The listing builds one solid part. Answer for the finished solid, in the listing's coordinates (mm). A direction names the side the tool comes from. Coordinates: 2 decimals unless noted, no trailing zeros. Loops run counter-clockwise (first coordinate to the right, second up) from the corner with the lowest first, then second, coordinate; pieces in that order, holes last. Notation, with made-up numbers: (-13.5, 24) - (42.5, 24) arc R35 cw to (42.5, 62) - close; hole circle Ø5 at (29.25, 21.25). An arc over 180 degrees is marked (long way). Return JSON: item names as keys, results as strings. Group by question number.
1. Each of these flat-tipped pins is pushed along its axis until it touches: P1, Ø4, axis at x = -6.5, y = -1.5, coming from the +Z side; P2, Ø1, axis at x = -4.5, y = -3.5, coming from the +Z side; P3, Ø3, axis at y = -1, z = -6.5, coming from the +X side (3 decimals). Where does it stop, or does it pass through?
2. Section B-B (z = 15.5) is taken. Write down the section's boundary in (x, y), and give its area (3 significant figures).
3. Find the intervals of material crossed by line 1 along Z through (x, y) = (2.5, -4.5); line 2 along Z through (x, y) = (-6.75, -6.5); line 3 along X through (y, z) = (-2.75, -3), in increasing order.
4. Which of the six approach directions +Z, -Z, +X, -X, +Y, -Y give full straight-line access (tool end or side, diameter ignored) to faces 1 (the face through (-1.037, -3.451, 14.204)), 2 (the face through (-8.336, -3.451, 16.078))?
5. Section C-C (x = 11.75) is taken. Write down the section's boundary in (y, z), and give its area (3 significant figures).
6. Section A-A (y = -2.75) is taken. Write down the section's boundary in (x, z) (3 decimals).
7. The mould has two halves that part along Z. Classify faces 3 (the face through (-0.07, 0, 10.03)), 4 (the face through (8.513, -3.451, 16.027)), 5 (the face through (-1.924, -3.465, -8.664)): pulls with the +Z half, pulls with the -Z half, needs draft (parallel to the pull), parting line crosses it, or undercut.
```python
from build123d import *

# Parameters (mm, degrees)
F0_R     = 8.875
F1_DEPTH = 7
F2_SIZE  = 1


with BuildPart() as f1:
    # F0 (on Front) → F1 (new body)
    with BuildSketch(Plane.XZ):
        with BuildLine():
            ThreePointArc((0, 10.625), (7.51301, 7.51301), (10.625, 0))
            Line((10.625, 0), (14.745765, 14.220767))
            Line((14.745765, 14.220767), (2.103486, 17.884132))
            Line((2.103486, 17.884132), (0, 10.625))
        make_face()
        with BuildLine():
            ThreePointArc((-10.625, 0), (-7.51301, 7.51301), (0, 10.625))
            Line((0, 10.625), (-2.103486, 17.884132))
            Line((-2.103486, 17.884132), (-14.745765, 14.220767))
            Line((-14.745765, 14.220767), (-10.625, 0))
        make_face()
        with BuildLine():
            ThreePointArc((-10.625, 0), (0, -10.625), (10.625, 0))
            ThreePointArc((10.625, 0), (7.51301, 7.51301), (0, 10.625))
            ThreePointArc((0, 10.625), (-7.51301, 7.51301), (-10.625, 0))
        make_face()
        Circle(F0_R, mode=Mode.SUBTRACT)
    extrude(amount=F1_DEPTH)

    # F2
    f2_edges = [f1.edges().sort_by_distance(p)[0] for p in [
        (-8.875, 0, 0),
        (-8.875, -7, 0),
    ]]
    chamfer(f2_edges, length=F2_SIZE)


solid = f1.part
```
The answers:
{
 "1": {"P1": "stops at z = 17.19", "P2": "stops at z = 17.33", "P3": "stops at x = 9.375"},
 "2": {"outline": "(-10.33, -7) - (-1.41, -7) - (-1.41, 0) - (-10.33, 0) - close; (1.41, -7) - (10.33, -7) - (10.33, 0) - (1.41, 0) - close", "area": "125 mm2"},
 "3": {"line 1": "z = -10.33 to -8.52, 8.52 to 17.77", "line 2": "z = -8.21 to -6.51, 6.51 to 16.54", "line 3": "x = -10.19 to -8.35, 8.35 to 10.19"},
 "4": {"face 1": "+Z, +Y, -Y", "face 2": "+Z, -X, +Y, -Y"},
 "5": {"outline": "(-7, 3.88) - (0, 3.88) - (0, 15.09) - (-7, 15.09) - close", "area": "78.4 mm2"},
 "6": {"outline": "(-14.746, 14.221) - (-10.625, 0) arc R10.625 ccw to (10.625, 0) - (14.746, 14.221) - (2.103, 17.884) - (0, 10.625) - (-2.103, 17.884) - close; hole circle Ø17.75 at (0, 0)"},
 "7": {"face 3": "needs draft", "face 4": "pulls with the +Z half", "face 5": "undercut"}
}
